Source: CAD feature listing. Evaluate the final solid. Frame: model axes, mm. Coordinates: 2 decimals unless noted, no trailing zeros. Write each loop counter-clockwise with the first axis right and the second up, starting at its lowest first coordinate (ties: lowest second). Pieces come first, ordered by that corner, then holes. Notation, with made-up numbers: (-24, -17) -> (2, -17) arc R15 ccw to (2, -1) -> close; hole circle Ø10 at (2.5, 36). An arc over 180 degrees is marked (long way). One line per item, written item: value. Start each with the question number.
1. Mould query, pull axis Y, two halves, no side actions, for faces 1 (the flat face through (6.172, -5, 0)), 2 (the cylindrical face through (-0.1, -0.75, 0.01)), 3 (the cylindrical face through (22.132, 23.809, 0.014)). Classes: released by +Y, released by -Y, zero draft, split by the parting line, or undercut.
2. Section query A-A, the plane z = -0.6. State how many separate pieces and enclosed holes the cut face has, and give its area (3 significant figures).
3. Section query C-C, the plane x = 19.25. Output: boundary loops of the cut face in (y, z).
4. Section query B-B, the plane y = -5. Output: boundary loops of the cut face in (x, z).
5. Line query: line 1 (Y direction, x = 1, z = -0.3); line 2 (Y direction, x = 0.5, z = 0.25); line 3 (X direction, y = 3.5, z = -0.7). Output: solid intervals per line, ascending.
6. First-contact query: P1, Ø0.6, axis at y = -8, z = 0, coming from the +X side; P2, Ø4, axis at x = 6.51, y = 13.13, coming from the +Z side. Flat tips, straight axial feed; report the tip coordinate or a pass-through.
from build123d import *

# Parameters (mm, degrees)
EXTRUDE_1_DEPTH     = 1
FILLET_1_R          = 5
SKETCH_2_R          = 1.6
CUT_EXTRUDE_1_DEPTH = 37.340563377


with BuildPart() as part:
    # ｽｹｯﾁ1 → ﾎﾞｽ - 押し出し1 (new, symmetric)
    with BuildSketch(Plane.XY):
        Polygon((-3.827856705, 2.446999561), (-3.827856705, -19.777202359), (6.172143295, -19.777202359), (6.172143295, 5.722797641), (24.203366215, 23.754020561), (17.132298403, 30.825088373), (-3.827856705, 9.864933264), align=None)
    extrude(amount=EXTRUDE_1_DEPTH, both=True)

    # ﾌｨﾚｯﾄ1
    fillet_1_edges = [part.edges().sort_by_distance(p)[0] for p in [
        (17.132298403, 30.825088373, 0),
        (-3.827856705, -19.777202359, 0),
        (6.172143295, -19.777202359, 0),
        (24.203366215, 23.754020561, 0),
    ]]
    fillet(fillet_1_edges, radius=FILLET_1_R - 0.0001)  # a hair under: the kernel refuses the full size

    # ｽｹｯﾁ2 → ｶｯﾄ - 押し出し1 (cut, through all)
    with BuildSketch(Plane.XY.offset(1)):
        with Locations((1.172143295, 0.222797641)):
            Circle(SKETCH_2_R)
        with Locations((1.172143295, -14.777202359)):
            Circle(SKETCH_2_R)
        with Locations((6.505160691, 13.126882849)):
            Circle(SKETCH_2_R)
        with Locations((17.111762409, 23.733484566)):
            Circle(SKETCH_2_R)
    extrude(amount=-CUT_EXTRUDE_1_DEPTH, mode=Mode.SUBTRACT)


solid = part.part
Computed values:
1. face 1: zero draft
1. face 2: undercut
1. face 3: split by the parting line
2. separate pieces: 1
2. enclosed holes: 4
2. area: 498 mm²
3. outline: (18.8, -1) -> (28.28, -1) -> (28.28, 1) -> (18.8, 1) -> close
4. outline: (-3.83, -1) -> (6.17, -1) -> (6.17, 1) -> (-3.83, 1) -> close
5. line 1: y = -19.77 to -16.37, -13.19 to -1.37, 1.81 to 14.69
5. line 2: y = -19.73 to -16.23, -13.33 to -1.23, 1.67 to 14.19
5. line 3: x = -3.83 to 6.17
6. P1: stops at x = 6.17
6. P2: stops at z = 1
